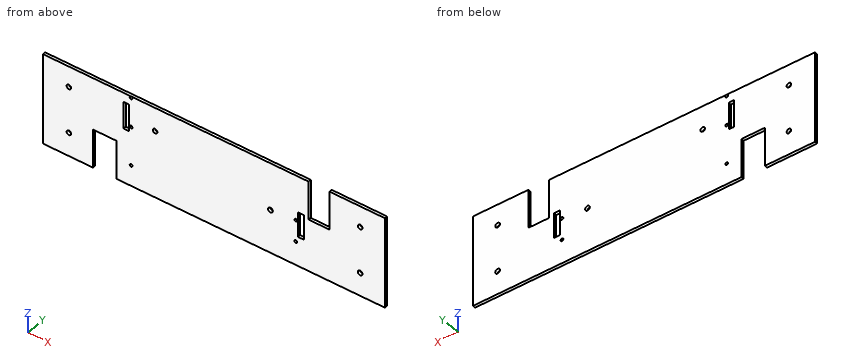
from build123d import *

# Parameters (mm, degrees)
SKETCH2_W           = 383.032
SKETCH2_H           = 101.6
BOSS_EXTRUDE1_DEPTH = 3.175
SKETCH3_R           = 2.54
SKETCH3_R_2         = 1.524
SKETCH3_W           = 26.128243683
SKETCH3_H           = 43.225676532
SKETCH3_W_2         = 6.096
SKETCH3_H_2         = 30.414908662
CUT_EXTRUDE1_DEPTH  = 5.08
SKETCH4_W           = 23.194024084
SKETCH4_H           = 43.199369669
SKETCH4_W_2         = 6.45398931
SKETCH4_H_2         = 28.034516067
SKETCH4_R           = 2.653649749
SKETCH4_R_2         = 2.61409985
SKETCH4_R_3         = 2.657297928
SKETCH4_R_4         = 1.524
CUT_EXTRUDE2_DEPTH  = 5.08
SKETCH5_W           = 11.780939099
SKETCH5_H           = 116.381398369
CUT_EXTRUDE3_DEPTH  = 6.35


with BuildPart() as part:
    # Sketch2 → Boss-Extrude1 (new body)
    with BuildSketch(Plane(origin=(0, 0, 0), x_dir=(1, 0, 0), z_dir=(0, 1, 0))):
        Rectangle(SKETCH2_W, SKETCH2_H)
    extrude(amount=BOSS_EXTRUDE1_DEPTH)

    # Sketch3 → Cut-Extrude1 (cut)
    with BuildSketch(Plane(origin=(0, 3.175, 0), x_dir=(1, 0, 0), z_dir=(0, 1, 0))):
        with Locations(Location((-160.218440268, 24.384, 0), (0, 0, 270))):
            Circle(SKETCH3_R)
        with Locations(Location((-160.218440268, -27.664005213, 0), (0, 0, 270))):
            Circle(SKETCH3_R)
        with Locations(Location((-90.932, -49.149, 0), (0, 0, 270))):
            Circle(SKETCH3_R_2)
        with Locations(Location((-90.932, -16.076263173, 0), (0, 0, 270))):
            Circle(SKETCH3_R_2)
        with Locations(Location((-90.932, 27.570881088, 0), (0, 0, 270))):
            Circle(SKETCH3_R_2)
        with Locations(Location((-64.2581016, -24.473600424, 0), (0, 0, 270))):
            Circle(SKETCH3_R)
        with Locations((-120.285878158, 29.187161734)):
            Rectangle(SKETCH3_W, SKETCH3_H)
        with Locations((-96.266, -25.392171491)):
            Rectangle(SKETCH3_W_2, SKETCH3_H_2)
    extrude(amount=-CUT_EXTRUDE1_DEPTH, mode=Mode.SUBTRACT)

    # Sketch4 → Cut-Extrude2 (cut)
    with BuildSketch(Plane(origin=(0, 3.175, 0), x_dir=(1, 0, 0), z_dir=(0, 1, 0))):
        with Locations((118.230976638, -29.200315166)):
            Rectangle(SKETCH4_W, SKETCH4_H)
        with Locations((98.119005345, 3.794694545)):
            Rectangle(SKETCH4_W_2, SKETCH4_H_2)
        with Locations(Location((164.103401606, 24.883919413, 0), (0, 0, 270))):
            Circle(SKETCH4_R)
        with Locations(Location((164.103401606, -27.372567953, 0), (0, 0, 270))):
            Circle(SKETCH4_R_2)
        with Locations(Location((64.135, 2.286, 0), (0, 0, 270))):
            Circle(SKETCH4_R_3)
        with Locations(Location((92.456, 24.257, 0), (0, 0, 270))):
            Circle(SKETCH4_R_4)
        with Locations(Location((92.456, 0, 0), (0, 0, 270))):
            Circle(SKETCH4_R_4)
    extrude(amount=-CUT_EXTRUDE2_DEPTH, mode=Mode.SUBTRACT)

    # Sketch5 → Cut-Extrude3 (cut)
    with BuildSketch(Plane(origin=(0, 3.175, 0), x_dir=(1, 0, 0), z_dir=(0, 1, 0))):
        with Locations((-194.920992361, 1.96348985)):
            Rectangle(SKETCH5_W, SKETCH5_H)
    extrude(amount=-CUT_EXTRUDE3_DEPTH, mode=Mode.SUBTRACT)


solid = part.part
CAD build for the part. Positions are in the model's coordinates, mm. Coordinates: 2 decimals unless noted, no trailing zeros. Loops run counter-clockwise (first coordinate to the right, second up) from the corner with the lowest first, then second, coordinate; pieces in that order, holes last. Notation, with made-up numbers: (20.25, 46.25) - (70.25, 46.25) arc R6 cw to (70.25, 54.25) - close; hole circle Ø10 at (-21, 76.5). An arc over 180 degrees is marked (long way). Write item = value, one per line. Start each with the question number.
Q1. Cut at B-B, the plane z = 34. List the corners of the cut face in (x, y) (3 decimals).
Q2. Cut at D-D, the plane x = 121. List the corners of the cut face in (y, z) (3 decimals), then the cut area to 3 significant figures.
Q3. Cut at A-A, the plane z = -43. List the corners of the cut face in (x, y) (3 decimals).
Q4. Flat gauge pin, fed straight in: pin 1 Ø1.6 at (x, y) = (120, 1) entering from +Z. Where does the tip first touch, or does it go through?
Q5. Cut at C-C, the plane y = 0.55. Give the number of separate pieces and of enclosed holes in the cut face, then the cut area to 3 significant figures.
Q6. Drill centre lines: L1, parallel to X at y = 0.1, z = 38; L2, parallel to X at y = 2.55, z = -10; L3, parallel to X at y = 2.2, z = 24.5. Where is each one in solid material? Low to high.
Computed:
q1.outline = (-189.031, 0) - (-99.314, 0) - (-99.314, 3.175) - (-189.031, 3.175) - close; (-93.218, 0) - (106.634, 0) - (106.634, 3.175) - (-93.218, 3.175) - close; (129.828, 0) - (191.516, 0) - (191.516, 3.175) - (129.828, 3.175) - close
q2.outline = (0, -50.8) - (3.175, -50.8) - (3.175, 7.601) - (0, 7.601) - close
q2.area = 185 mm²
q3.outline = (-189.031, 0) - (-133.35, 0) - (-133.35, 3.175) - (-189.031, 3.175) - close; (-107.222, 0) - (191.516, 0) - (191.516, 3.175) - (-107.222, 3.175) - close
q4.pin_1 = 7.6
q5.separate_pieces = 1
q5.enclosed_holes = 13
q5.area = 36,000 mm²
q6.L1 = -189.03 to -99.31, -93.22 to 106.63, 129.83 to 191.52
q6.L2 = -189.03 to -133.35, -107.22 to 94.89, 101.35 to 191.52
q6.L3 = -189.03 to -99.31, -93.22 to -66.8, -61.72 to 106.63, 129.83 to 191.52
